from build123d import *

# Parameters (mm, degrees)
SKETCH_1_W      = 105
SKETCH_1_H      = 20
SKETCH_1_R      = 1.6
SKETCH_1_R_2    = 2.25
EXTRUDE_1_DEPTH = 5
FILLET_2_R      = 5
CHAMFER_1_SIZE  = 1
CHAMFER_2_SIZE  = 1


with BuildPart() as part:
    # Эскиз1 → Бобышка-Вытянуть1 (new body)
    with BuildSketch(Plane(origin=(0, 0, 0), x_dir=(1, 0, 0), z_dir=(0, 1, 0))):
        with Locations((52.5, 10)):
            Rectangle(SKETCH_1_W, SKETCH_1_H)
        with Locations((19, 10)):
            Circle(SKETCH_1_R, mode=Mode.SUBTRACT)
        with Locations((86, 10)):
            Circle(SKETCH_1_R, mode=Mode.SUBTRACT)
        with Locations((7, 10)):
            Circle(SKETCH_1_R_2, mode=Mode.SUBTRACT)
        with Locations((98, 10)):
            Circle(SKETCH_1_R_2, mode=Mode.SUBTRACT)
    extrude(amount=EXTRUDE_1_DEPTH)

    # Скругление2
    fillet_2_edges = [part.edges().sort_by_distance(p)[0] for p in [
        (0, 2.5, -20),
        (105, 2.5, -20),
        (105, 2.5, 0),
        (0, 2.5, 0),
    ]]
    fillet(fillet_2_edges, radius=FILLET_2_R)

    # Фаска1
    chamfer_1_edges = [part.edges().sort_by_distance(p)[0] for p in [
        (4.75, 5, -10),
        (95.75, 5, -10),
    ]]
    chamfer(chamfer_1_edges, length=CHAMFER_1_SIZE)

    # Фаска2
    chamfer_2_edges = [part.edges().sort_by_distance(p)[0] for p in [
        (17.4, 0, -10),
        (84.4, 0, -10),
    ]]
    chamfer(chamfer_2_edges, length=CHAMFER_2_SIZE)


solid = part.part
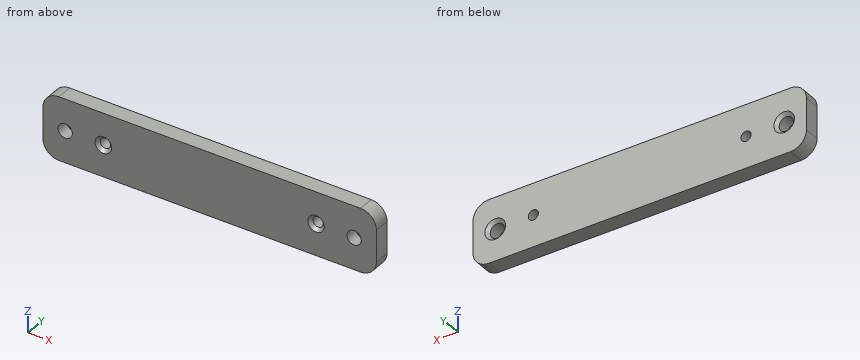
Geometry check sheet. Reference: the model listing, model coordinates, mm. Round coordinates to 2 decimals unless told otherwise and drop trailing zeros. Order: outer loops, then holes, each group sorted by start corner. A loop starts at its lowest first (then second) coordinate and runs counter-clockwise, first axis right, second up. Notation, with made-up numbers: (17.5, -36) -> (72.5, -36) arc R14 ccw to (72.5, -21) -> close; hole circle Ø10 at (45, 22.25). An arc over 180 degrees is marked (long way). Use one line per item in the form item = value.
1. Cross-section at B-B, the plane x = 7. Enter the section's corners in (y, z), plus the area to 3 significant figures.
Working result:
outline = (0, -20) -> (5, -20) -> (5, -13.25) -> (4, -12.25) -> (0, -12.25) -> close; (0, -7.75) -> (4, -7.75) -> (5, -6.75) -> (5, 0) -> (0, 0) -> close
area = 76.5 mm^2
2. Scan lines: line 1 along X through (y, z) = (1.6, -10); line 2 along Z through (x, y) = (86, 3.2); line 3 along X through (y, z) = (4.05, -10). Record each from-to range of solid material in increasing order. Write a range as from..to.
Working result:
line_1 = 0..4.75, 9.25..17.4, 20.6..84.4, 87.6..95.75, 100.25..105
line_2 = -20..-11.6, -8.4..0
line_3 = 0..4.7, 9.3..17.4, 20.6..84.4, 87.6..95.7, 100.3..105
3. Cross-section at A-A, the plane z = -10. Enter the section's corners in (x, y), plus the area to 3 significant figures.
Working result:
outline = (0, 0) -> (4.75, 0) -> (4.75, 4) -> (3.75, 5) -> (0, 5) -> close; (9.25, 0) -> (16.4, 0) -> (17.4, 1) -> (17.4, 5) -> (10.25, 5) -> (9.25, 4) -> close; (20.6, 1) -> (21.6, 0) -> (83.4, 0) -> (84.4, 1) -> (84.4, 5) -> (20.6, 5) -> close; (87.6, 1) -> (88.6, 0) -> (95.75, 0) -> (95.75, 4) -> (94.75, 5) -> (87.6, 5) -> close; (100.25, 0) -> (105, 0) -> (105, 5) -> (101.25, 5) -> (100.25, 4) -> close
area = 444 mm^2
4. Cross-section at C-C, the plane x = 19. Enter the section's corners in (y, z).
Working result:
outline = (0, -20) -> (5, -20) -> (5, -11.6) -> (1, -11.6) -> (0, -12.6) -> close; (0, -7.4) -> (1, -8.4) -> (5, -8.4) -> (5, 0) -> (0, 0) -> close
5. Go/stop test with a flat-tipped pin: pin 1 (3.5 mm diameter, centred on x = 98, z = -10, fed in from +Y). Record where the tip stops, or that it passes through.
Working result:
pin_1 = through
